Geometry check sheet. Reference: the model listing, model coordinates, mm. A direction names the side the tool comes from. Round coordinates to 2 decimals unless told otherwise and drop trailing zeros. Order: outer loops, then holes, each group sorted by start corner. A loop starts at its lowest first (then second) coordinate and runs counter-clockwise, first axis right, second up. Notation, with made-up numbers: (-12.5, 38.25) -> (12.5, 38.25) arc R14 cw to (12.5, 64.25) -> close; hole circle Ø5 at (-40, 83.5). An arc over 180 degrees is marked (long way). Use a Markdown table: item, result. Add a question column.
Item 1: Gauge pin test, flat ends, axial feed: pin 1 Ø3 at (x, z) = (35.5, -1.5) entering from +Y; pin 2 Ø15.5 at (y, z) = (23.5, 23.5) entering from -X; pin 3 Ø6 at (y, z) = (30.5, 3) entering from -X; pin 4 Ø10 at (x, y) = (19, 18.5) entering from -Z. Record the tip position at first contact, or that the pin passes through.
Item 2: Sectioned sample at A-A, the plane x = -55.5. Record the cut outline in (y, z).
Item 3: Material ranges on probe 1 along X at (y, z) = (60.3, 38.5); probe 2 along X at (y, z) = (59.7, -38.5); probe 3 along X at (y, z) = (4.5, -43), recorded low to high. Write a range as [from, to].
Item 4: Set-up check for faces 1 (the flat face through (38, 1, -5)), 2 (the flat face through (39.5, 8, 15)), 3 (the flat face through (-48, 29, 7.7)), 4 (the flat face through (-41, 7, 27.5)): record each of +Z, -Z, +X, -X, +Y, -Y from which the full face is reachable in a straight line by a thin tool's end or side.
Item 5: Sectioned sample at C-C, the plane z = 13. Record the cut outline in (x, y).
Item 6: Mould release check, pull along X, two halves, no side actions. Record for faces 5 (the flat face through (36, 6, 42.5)), 6 (the cylindrical face through (53.84, 59.48, -36.98)), 7 (the flat face through (-2.5, 5, -47)), 8 (the flat face through (52.5, 29, 15)): pulls with the +X half, pulls with the -X half, needs draft (parallel to the pull), parting line crosses it, or undercut.
Item 7: Sectioned sample at D-D, the plane z = -38.5. Record the cut outline in (x, y), and give its area (3 significant figures).
Item 8: Sectioned sample at B-B, the plane y = 19.5. Record the cut outline in (x, z), and give its area (3 significant figures).
Autodesk Inventor part; units mm, degrees
ref_plane "YZ Plane" through (0, 0, 0) normal (1, 0, 0) x (0, 1, 0)
ref_plane "XZ Plane" through (0, 0, 0) normal (0, 1, 0) x (-1, 0, 0)
ref_plane "XY Plane" through (0, 0, 0) normal (0, 0, 1) x (1, 0, 0)
sketch "Boceto1" plane through (0, 0, 0) normal (0, 1, 0) x (-1, 0, 0)
  line L0 (39.5, 42.5) -> (-39.5, 42.5)
  line L1 (-39.5, 42.5) -> (-39.5, -42.5)
  line L2 (-39.5, -42.5) -> (39.5, -42.5)
  line L3 (39.5, -42.5) -> (39.5, 42.5)
  line L4 (39.5, 42.5) -> (-39.5, -42.5) construction
  line L5 (-39.5, 42.5) -> (39.5, -42.5) construction
  line L6 (42.5, 45.5) -> (-42.5, 45.5)
  line L7 (-42.5, 45.5) -> (-42.5, -45.5)
  line L8 (-42.5, -45.5) -> (42.5, -45.5)
  line L9 (42.5, -45.5) -> (42.5, 45.5)
  point P0 (0, 0)
  point P1 (0, 0)
  dimension "d0" = 79
  dimension "d1" = 85
  dimension "d2" = 3
extrude "Extrusión1" add sketch "Boceto1" along normal blind 10 contours L3 L2 L1 L0 | L9 L8 L7 L6
sketch "Boceto2" plane through (0, 10, 0) normal (0, 1, 0) x (1, 0, 0)
  line L0 (-42.5, 45.5) -> (-42.5, -45.5)
  line L1 (42.5, -45.5) -> (-42.5, -45.5)
  line L2 (-42.5, -45.5) -> (-42.5, 45.5)
  line L3 (-42.5, 45.5) -> (42.5, 45.5)
  line L4 (42.5, 45.5) -> (42.5, -45.5)
  line L5 (42.5, -45.5) -> (-42.5, 45.5) construction
  line L6 (-42.5, -45.5) -> (42.5, 45.5) construction
  line L7 (-39.5, -42.5) -> (39.5, -42.5)
  line L8 (39.5, -42.5) -> (39.5, 42.5)
  line L9 (39.5, 42.5) -> (-39.5, 42.5)
  line L10 (-39.5, 42.5) -> (-39.5, -42.5)
  line L11 (0, -42.5) -> (0, -45.5)
  line L12 (-42.5, -45.5) -> (42.5, -45.5)
  line L13 (-15, -45.5) -> (15, -45.5)
  line L14 (15, -45.5) -> (15, -42.5)
  line L15 (15, -42.5) -> (-15, -42.5)
  line L16 (-15, -42.5) -> (-15, -45.5)
  line L17 (-15, -45.5) -> (15, -42.5) construction
  line L18 (15, -45.5) -> (-15, -42.5) construction
  line L19 (-65.3363, 15.3) -> (96.4695, 15.3)
  point P0 (0, 0)
  point P1 (0, -44)
  point P2 (39.5, 15.3)
  point P3 (-39.5, 15.3)
  dimension "d8" = 3
  dimension "d9" = 85
  dimension "d10" = 79
  dimension "d11" = 30
  dimension "d12" = 57.8
extrude "Extrusión2" cut sketch "Boceto2" against normal blind 5 contours L19 L8 L7 L10
sketch "Boceto3" plane through (0, 0, 0) normal (0, 1, 0) x (-1, 0, 0)
  line L0 (-42.5, 45.5) -> (-42.5, -15.3)
  line L1 (42.5, -45.5) -> (-42.5, -45.5)
  line L2 (-42.5, -45.5) -> (-42.5, -15.3)
  line L3 (-42.5, -15.3) -> (42.5, -15.3)
  line L4 (42.5, -15.3) -> (42.5, -45.5)
  line L5 (-45.5, -48.5) -> (45.5, -48.5)
  line L6 (45.5, -48.5) -> (45.5, -12.3)
  line L7 (45.5, -12.3) -> (-45.5, -12.3)
  line L8 (-45.5, -12.3) -> (-45.5, -48.5)
  line L9 (45.5, -15.3) -> (-45.5, -15.3)
  line L10 (-12.5, -48.5) -> (-12.5, -45.5)
  line L11 (-42.5, -45.5) -> (42.5, -45.5)
  line L12 (42.5, -45.5) -> (42.5, -48.5)
  line L13 (42.5, -15.3) -> (42.5, -12.3)
  line L14 (42.5, -45.5) -> (42.5, 45.5)
  line L15 (-42.5, -15.3) -> (-42.5, -12.3)
  line L16 (-42.5, 45.5) -> (-42.5, -45.5)
  line L17 (-42.5, -45.5) -> (-42.5, -48.5)
  line L18 (-42.5, -45.5) -> (42.5, -45.5)
  line L19 (2.5, -48.5) -> (32.5, -48.5)
  line L20 (32.5, -48.5) -> (32.5, -45.5)
  line L21 (32.5, -45.5) -> (2.5, -45.5)
  line L22 (2.5, -45.5) -> (2.5, -48.5)
  point P0 (0, 0)
  point P1 (0, 0)
  point P2 (-12.5, -47)
  point P3 (2.5, -45.5)
  point P4 (42.5, -47)
  point P5 (32.5, -47)
  dimension "d15" = 3
  dimension "d16" = 30
  dimension "d21" = 30
  dimension "d24" = 10
extrude "Extrusión3" add sketch "Boceto3" along normal blind 10 contours L7 L13 L3 L0 | L0 L9 L8 L7 | L3 L4 L1 L2 | L2 L17 L5 L8 L9 | L7 L6 L9 L13 | L9 L6 L5 L12 L4 | L1 L20 L5 L22
sketch "Boceto4" plane through (0, 10, 0) normal (0, 1, 0) x (1, 0, 0)
  line L0 (-39.5, 15.3) -> (39.5, 15.3)
  line L1 (0, 15.3) -> (0, 45.5)
  line L2 (42.5, 45.5) -> (-42.5, 45.5)
  line L3 (-42.5, 45.5) -> (42.5, 45.5)
  line L4 (42.5, 45.5) -> (42.5, 15.3)
  line L5 (42.5, 15.3) -> (-42.5, 15.3)
  line L6 (-42.5, 15.3) -> (-42.5, 45.5)
  line L7 (-42.5, 45.5) -> (42.5, 15.3) construction
  line L8 (42.5, 45.5) -> (-42.5, 15.3) construction
  point P0 (0, 0)
  point P1 (0, 0)
  point P2 (0, 30.4)
extrude "Extrusión4" cut sketch "Boceto4" against normal blind 8
sketch "Boceto5" plane through (-42.5, 0, 45.5) normal (-1, 0, 0) x (0, 0, 1)
  line L0 (-18, 10) -> (-28, 10)
  line L1 (-28, 10) -> (-28, 5)
  line L2 (-28, 5) -> (-18, 5)
  line L3 (-18, 5) -> (-18, 10)
  line L4 (-3, 5) -> (-57.8, 5)
  line L5 (-3, 10) -> (-3, 5)
  line L6 (-57.8, 10) -> (0, 10)
  point P0 (-45.5, 0)
  point P1 (-23, 5)
  dimension "d25" = 10
  dimension "d27" = 15
  dimension "d28" = 0
  dimension "d29" = 0
extrude "Extrusión5" cut sketch "Boceto5" against normal blind 10 contours L3 L2 L1 L0
sketch "Boceto6" plane through (-42.5, 0, 45.5) normal (0, 0, 1) x (1, 0, 0)
  line L0 (67, 5) -> (57, 5)
  line L1 (57, 5) -> (57, 10)
  line L2 (57, 10) -> (67, 10)
  line L3 (67, 10) -> (67, 5)
  line L4 (82, 5) -> (3, 5)
  line L5 (85, 0) -> (85, 10)
  line L6 (0, 10) -> (85, 10)
  point P0 (42.5, 0)
  point P1 (62, 5)
  dimension "d32" = 10
  dimension "d33" = 18
  dimension "d34" = 0
  dimension "d35" = 0
extrude "Extrusión6" cut sketch "Boceto6" against normal blind 10
sketch "Boceto7" plane through (42.5, 0, 45.5) normal (1, 0, 0) x (0, 0, -1)
  line L0 (57.8, 10) -> (3, 10)
  line L1 (3, 10) -> (18, 10)
  line L2 (18, 10) -> (18, 1)
  line L3 (18, 1) -> (3, 1)
  line L4 (3, 1) -> (3, 10)
  line L5 (3, 10) -> (3, 5)
  line L6 (57.8, 10) -> (28, 10)
  line L7 (57.8, 10) -> (42.8, 10)
  line L8 (42.8, 10) -> (42.8, 1)
  line L9 (42.8, 1) -> (57.8, 1)
  line L10 (57.8, 1) -> (57.8, 10)
  point P0 (45.5, 0)
  point P1 (0, 10)
  dimension "d41" = 15
  dimension "d42" = 9
  dimension "d43" = 0
  dimension "d46" = 15
  dimension "d47" = 9
extrude "Extrusión7" cut sketch "Boceto7" against normal blind 10
sketch "Boceto8" plane through (0, 0, 0) normal (0, 1, 0) x (-1, 0, 0)
  line L0 (42.5, -12.3) -> (42.5, 45.5)
  line L1 (42.5, -12.3) -> (52.5, -12.3)
  line L2 (52.5, -12.3) -> (52.5, 7.7)
  line L3 (52.5, 7.7) -> (42.5, 7.7)
  line L4 (42.5, 7.7) -> (42.5, -12.3)
  line L5 (45.5, -12.3) -> (42.5, -12.3)
  line L6 (-42.5, 45.5) -> (-42.5, -12.3)
  line L7 (-42.5, 5.1) -> (-52.5, 5.1)
  line L8 (-52.5, 5.1) -> (-52.5, 25.1)
  line L9 (-52.5, 25.1) -> (-42.5, 25.1)
  line L10 (-42.5, 25.1) -> (-42.5, 5.1)
  line L11 (-42.5, 2.7) -> (-39.5, 2.7)
  line L12 (-39.5, 27.5) -> (-42.5, 27.5)
  point P0 (0, 0)
  dimension "d48" = 10
  dimension "d49" = 20
  dimension "d50" = 0
  dimension "d51" = 10
  dimension "d52" = 20
  dimension "d53" = 2.4
  dimension "d54" = 2.4
extrude "Extrusión8" add sketch "Boceto8" along normal blind 58
sketch "Boceto9" plane through (0, 58, 0) normal (0, 1, 0) x (1, 0, 0)
  line L0 (-69.4566, 48.5) -> (100.0188, 48.5)
  line L1 (45.5, 48.5) -> (12.5, 48.5)
  line L2 (-42.5, -45.5) -> (42.5, -45.5)
  line L3 (-42.5, -45.5) -> (-83.2167, -45.5)
  line L4 (-83.2167, -45.5) -> (109.2502, -45.5)
  line L5 (65.5, 48.5) -> (65.5, -45.5)
  line L6 (45.5, 12.3) -> (45.5, 48.5)
  circle A0 centre (55.5, 38.5) radius 2.25
  line L7 (65.5, 0) -> (100.0188, 0)
  circle A1 centre (55.5, -38.5) radius 2.25
  line L8 (0, -45.5) -> (0, -59.2916)
  line L9 (-65.5, 48.5) -> (-65.5, -45.5)
  circle A2 centre (-55.5, -38.5) radius 2.25
  circle A3 centre (-55.5, 38.5) radius 2.25
  line L10 (-42.5, 12.3) -> (-42.5, -45.5)
  line L11 (-42.5, -45.5) -> (-42.5, 12.3)
  line L12 (-45.5, 12.3) -> (-42.5, 12.3)
  line L13 (-42.5, 12.3) -> (-45.5, 12.3)
  line L14 (-45.5, 48.5) -> (-45.5, 12.3)
  line L15 (-45.5, 12.3) -> (-45.5, 48.5)
  line L16 (-45.5, 48.5) -> (-65.5, 48.5)
  line L17 (42.5, 12.3) -> (45.5, 12.3)
  line L18 (45.5, 48.5) -> (45.5, 12.3)
  line L19 (45.5, 12.3) -> (42.5, 12.3)
  line L20 (15, -45.5) -> (42.5, -45.5)
  line L21 (42.5, 12.3) -> (42.5, -45.5)
  line L22 (42.5, -45.5) -> (65.5, -45.5)
  point P0 (0, 0)
  point P1 (0, 0)
  dimension "d57" = 20
  dimension "d58" = 4.5
  dimension "d59" = 10
  dimension "d60" = 10
extrude "Extrusión9" add sketch "Boceto9" along normal blind 3 contours L0 L14 L12 L10 L3 L9 | L0 L5 L4 L21 L17 L6
properties part number "batter_pack_top"
Found:
| question | item | result |
|---|---|---|
| 1 | pin 1 | stops at y = 1 |
| 1 | pin 2 | stops at x = 42.5 |
| 1 | pin 3 | stops at x = -52.5 |
| 1 | pin 4 | passes through |
| 2 | outline | (58, -48.5) -> (61, -48.5) -> (61, -40.75) -> (58, -40.75) -> close; (58, -36.25) -> (61, -36.25) -> (61, 36.25) -> (58, 36.25) -> close; (58, 40.75) -> (61, 40.75) -> (61, 45.5) -> (58, 45.5) -> close |
| 3 | probe 1 | x = [-65.5, -57.75], [-53.25, -42.5], [42.5, 53.25], [57.75, 65.5] |
| 3 | probe 2 | x = [-65.5, -57.75], [-53.25, -45.5], [45.5, 53.25], [57.75, 65.5] |
| 3 | probe 3 | x = [-45.5, -42.5], [42.5, 45.5] |
| 4 | face 1 | +X, +Y |
| 4 | face 2 | +Y |
| 4 | face 3 | +Z, -X, -Y |
| 4 | face 4 | -X, +Y |
| 5 | outline | (-65.5, 58) -> (-42.5, 58) -> (-42.5, 61) -> (-65.5, 61) -> close; (-42.5, 0) -> (52.5, 0) -> (52.5, 58) -> (65.5, 58) -> (65.5, 61) -> (42.5, 61) -> (42.5, 10) -> (39.5, 10) -> (39.5, 5) -> (-39.5, 5) -> (-39.5, 10) -> (-42.5, 10) -> close |
| 6 | face 5 | needs draft |
| 6 | face 6 | undercut |
| 6 | face 7 | undercut |
| 6 | face 8 | pulls with the +X half |
| 7 | outline | (-65.5, 58) -> (-57.75, 58) -> (-57.75, 61) -> (-65.5, 61) -> close; (-53.25, 58) -> (-45.5, 58) -> (-45.5, 61) -> (-53.25, 61) -> close; (-45.5, 0) -> (45.5, 0) -> (45.5, 10) -> (42.5, 10) -> (42.5, 2) -> (-42.5, 2) -> (-42.5, 10) -> (-45.5, 10) -> close; (45.5, 58) -> (53.25, 58) -> (53.25, 61) -> (45.5, 61) -> close; (57.75, 58) -> (65.5, 58) -> (65.5, 61) -> (57.75, 61) -> close |
| 7 | area | 323 mm2 |
| 8 | outline | (-52.5, -12.3) -> (-42.5, -12.3) -> (-42.5, 7.7) -> (-52.5, 7.7) -> close; (42.5, 5.1) -> (52.5, 5.1) -> (52.5, 25.1) -> (42.5, 25.1) -> close |
| 8 | area | 400 mm2 |
